Can you work these out from the model? Positions are in its coordinate system, mm. A direction names the side the tool comes from. Give positions to 0.01 mm unless a question says otherwise; leave off trailing zeros. Write each loop counter-clockwise with the first axis right and the second up, starting at its lowest first coordinate (ties: lowest second). Pieces come first, ordered by that corner, then holes. Notation, with made-up numbers: (67, 50) -> (90, 50) arc R12 cw to (90, 67) -> close; hole circle Ø2 at (-28, 24). An arc over 180 degrees is marked (long way). Answer as CSV lines item,"result". Start each with the question number.
1. I need wall thicknesses on line 1 (Y direction, x = -26, z = 16.5); line 2 (Z direction, x = 7.5, y = -45); line 3 (Y direction, x = 3, z = -12.5). Which ranges of each line are inside material? Lowest first, please. Write a range as [from, to].
2. If we section it at C-C on y = -20.5: Write out the boundary of the cut face in (x, z), plus the area to 3 significant figures.
3. If we section it at B-B on z = 2: Write out the boundary of the cut face in (x, y).
4. If we section it at A-A on x = 0: Write out the boundary of the cut face in (y, z), plus the area to 3 significant figures.
5. I'm going to push flat-ended pins straight in: P1, Ø3, axis at y = -26, z = -6.5, coming from the -X side; P2, Ø2, axis at x = -7.5, z = 22.5, coming from the -Y side; P3, Ø20, axis at x = -11.5, y = -18.5, coming from the +Z side; P4, Ø6, axis at x = -33.5, y = -26.5, coming from the +Z side. Where does each tip first touch, or does it pass through?
6. On a 3-axis mill with a long thin cutter (end or side, diameter ignored), from which of +Z, -Z, +X, -X, +Y, -Y can I reach the whole of each face in a straight line? I mean faces 1 (the face through (5, -25, 2)), 2 (the face through (-1, 0, 0)). Say none if no direction works.
7. If we section it at D-D on z = 9: Write out the boundary of the cut face in (x, y), plus the area to 3 significant figures.
```python
from build123d import *

# Parameters (mm, degrees)
F0_W     = 80
F0_H     = 65
F1_DEPTH = 55
F2_W     = 70
F2_H     = 45
F3_DEPTH = 10
F4_W     = 70
F4_H     = 15
F5_DEPTH = 45
F7_DEPTH = 30


with BuildPart() as f1:
    # F0 (on Front) → F1 (new body)
    with BuildSketch(Plane.XZ):
        Rectangle(F0_W, F0_H)
    extrude(amount=F1_DEPTH)

    # F2 (on face) → F3 (cut)
    with BuildSketch(Plane.XY.offset(32.5)):
        with Locations((-5, -32.5)):
            Rectangle(F2_W, F2_H)
    extrude(amount=-F3_DEPTH, mode=Mode.SUBTRACT)

    # F4 (on face) → F5 (cut)
    with BuildSketch(Plane.XY.offset(22.5)):
        with Locations((-5, -47.5)):
            Rectangle(F4_W, F4_H)
    extrude(amount=-F5_DEPTH, mode=Mode.SUBTRACT)

    # F6 (on face) → F7 (cut)
    with BuildSketch(Plane.XZ.offset(40)):
        Polygon((-40, 22.5), (-40, -12.5), (-20, -12.5), (-20, -2.5), (5, -2.5), (5, 7.5), (30, 7.5), (30, 22.5), align=None)
    extrude(amount=-F7_DEPTH, mode=Mode.SUBTRACT)


solid = f1.part
```
Computed values:
1,line 1,"y = [-10, 0]"
1,line 2,"z = [-32.5, -22.5]"
1,line 3,"y = [-40, 0]"
2,outline,"(-40, -32.5) -> (40, -32.5) -> (40, 32.5) -> (30, 32.5) -> (30, 7.5) -> (5, 7.5) -> (5, -2.5) -> (-20, -2.5) -> (-20, -12.5) -> (-40, -12.5) -> close"
2,area,"2,800 mm2"
3,outline,"(-40, -10) -> (5, -10) -> (5, -40) -> (30, -40) -> (30, -55) -> (40, -55) -> (40, 0) -> (-40, 0) -> close"
4,outline,"(-55, -32.5) -> (0, -32.5) -> (0, 32.5) -> (-10, 32.5) -> (-10, -2.5) -> (-40, -2.5) -> (-40, -22.5) -> (-55, -22.5) -> close"
4,area,"1,700 mm2"
5,P1,"stops at x = -20"
5,P2,"stops at y = -10"
5,P3,"stops at z = 32.5"
5,P4,"stops at z = -12.5"
6,face 1,"+Z, -X, -Y"
6,face 2,"+Z, -Z, +X, -X, +Y"
7,outline,"(-40, -10) -> (30, -10) -> (30, -55) -> (40, -55) -> (40, 0) -> (-40, 0) -> close"
7,area,"1,250 mm2"
